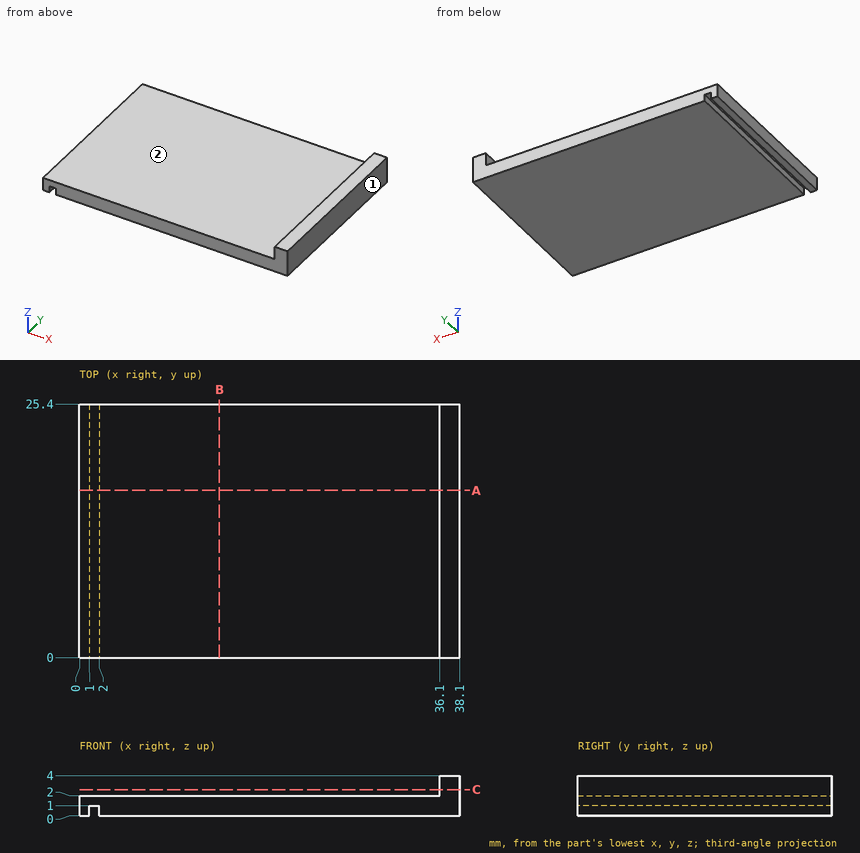
Input: dimensioned drawing with shaded views. Units: mm. Origin: part minimum x, y, z. A direction names the side the tool comes from. Coordinates: 2 decimals unless noted, no trailing zeros. Write each loop counter-clockwise with the first axis right and the second up, starting at its lowest first coordinate (ties: lowest second). Pieces come first, ordered by that corner, then holes. Notation, with made-up numbers: M 20.5,-5.5 L 73.5,-5.5 A29 cw 73.5,31.5 Z; hole C -22,71 d11. An arc over 180 degrees is marked long. Answer as CSV lines item,"result". Start each with the question number.
Q1. Cut plane B-B on x = 14. Return the cut outline in (y, z).
Q2. Pin query (flat end, axial travel): P1, Ø12, axis at x = 9.5, y = 11, coming from the +Z side; P2, Ø0.5, axis at x = 1.5, y = 13, coming from the -Z side; P3, Ø1.6, axis at y = 12.5, z = 3.5, coming from the -X side. Return the tip coordinate at first contact, or that it passes through.
Q3. Cut plane A-A on y = 16.75. Return the cut outline in (x, z), then the cut area to 3 significant figures.
Q4. Cut plane C-C on z = 2.6. Return the cut outline in (x, y), then the cut area to 3 significant figures.
Q5. Reachability of the marked faces 1 and 2 from +Z, -Z, +X, -X, +Y, -Y: full face, straight path, thin tool, end or side. Return the list, or none.
Q6. Line query: line 1 (X direction, y = 10.5, z = 0.9); line 2 (X direction, y = 23.5, z = 3.45); line 3 (Z direction, x = 30, y = 11.25). Output: solid intervals per line, ascending. Write a range as from..to.
Findings below:
1,outline,"M 0,0 L 25.4,0 L 25.4,2 L 0,2 Z"
2,P1,"stops at z = 2"
2,P2,"stops at z = 1"
2,P3,"stops at x = 36.1"
3,outline,"M 0,0 L 1,0 L 1,1 L 2,1 L 2,0 L 38.1,0 L 38.1,4 L 36.1,4 L 36.1,2 L 0,2 Z"
3,area,"79.2 mm2"
4,outline,"M 36.1,0 L 38.1,0 L 38.1,25.4 L 36.1,25.4 Z"
4,area,"50.8 mm2"
5,face 1,"+Z, -Z, +X, +Y, -Y"
5,face 2,"+Z, -X, +Y, -Y"
6,line 1,"x = 0..1, 2..38.1"
6,line 2,"x = 36.1..38.1"
6,line 3,"z = 0..2"
